```python
from build123d import *

# Parameters (mm, degrees)
F0_R      = 2.5
F1_DEPTH  = 2
F12_DEPTH = 2.0010001


with BuildPart() as f1:
    # F0 (on Top) → F1 (new body)
    with BuildSketch(Plane.XY):
        Polygon((-9.1669032276, 25.6), (-19.9169032276, 25.6), (-19.9169032276, 0), (-9.1669032276, 0), (-1.5169032276, 7.9), (30.5230967724, 7.9), (30.5230967724, 16.4), (2.6230967724, 16.4), (2.6230967724, 18.7), (-1.5169032276, 18.7), align=None)
        with Locations((-15.3946050969, 12.8)):
            Circle(F0_R, mode=Mode.SUBTRACT)
    extrude(amount=F1_DEPTH)

    # F4: sweep along a path in F2
    with BuildLine(Plane.XY.offset(2)) as f4_path:
        Line((2.6230967724, 15.15), (30.5230967724, 15.15))
    # F3 (on face) → F4 (sweep, cut)
    with BuildSketch(Plane.YZ.offset(2.6230967724)):
        with BuildLine():
            Line((17.3, 2), (15.3, 2))
            Line((15.3, 2), (14.7, 2))
            Line((14.7, 2), (15.5823529412, 0.75))
            add(Edge.make_bspline(
                [(15.5823529412, 0.75), (16.5972711165, 1.727867192), (16.3149181753, 1.727867192), (17.3, 2)],
                knots=[0, 0, 0, 0, 2.1243378777, 2.1243378777, 2.1243378777, 2.1243378777], degree=3))
        make_face()
    sweep(path=f4_path.line, mode=Mode.SUBTRACT)

    # F7: sweep along a path in F5
    with BuildLine(Plane.XY.offset(2)) as f7_path:
        Line((2.6230967724, 10.25), (30.5230967724, 10.25))
    # F6 (on face) → F7 (sweep, cut)
    with BuildSketch(Plane.YZ.offset(2.6230967724)):
        with BuildLine():
            add(Edge.make_bspline(
                [(11.55, 2), (11.1790336668, 1.9353309371), (10.4687979638, 0.1254777743), (8.7644318119, 0.7537172832), (8.7, 2)],
                knots=[0, 0, 0, 0, 0.4876224091, 1, 1, 1, 1], degree=3))
            Line((11.55, 2), (8.7, 2))
        make_face()
    sweep(path=f7_path.line, mode=Mode.SUBTRACT)

    # F10: sweep along a path in F8
    with BuildLine(Plane(origin=(0, 0, 0), x_dir=(1, 0, 0), z_dir=(0, 0, -1))) as f10_path:
        Line((2.6230967724, -17.2), (30.5230967724, -17.2))
    # F9 (on face) → F10 (sweep, cut)
    with BuildSketch(Plane.YZ.offset(2.6230967724)):
        with BuildLine():
            Line((17.2, 0), (17.2, 1))
            add(Edge.make_bspline(
                [(17.2, 1), (16.4, 1), (16.0935369316, 1.4085311701), (15.3480378536, 0.0682215952), (14.85, 0)],
                knots=[0, 0, 0, 0, 0.2283467357, 0.4887534963, 0.4887534963, 0.4887534963, 0.4887534963], degree=3))
            Line((14.85, 0), (17.2, 0))
        make_face()
        with BuildLine():
            Line((12.35, 0), (14.6790269663, 0))
            add(Edge.make_bspline(
                [(14.6790269663, 0), (14.1576409549, 0.0644703918), (13.0556896692, 1.1783434405), (12.4299004674, 0.6828821497), (12.35, 0)],
                knots=[0.5179423028, 0.5179423028, 0.5179423028, 0.5179423028, 0.7800763138, 1, 1, 1, 1], degree=3))
        make_face()
        with BuildLine():
            add(Edge.make_bspline(
                [(14.85, 0), (14.7941752951, -0.0076469096), (14.7370836655, -0.0071788235), (14.6790269663, 0)],
                knots=[0.4887534963, 0.4887534963, 0.4887534963, 0.4887534963, 0.5179423028, 0.5179423028, 0.5179423028, 0.5179423028], degree=3))
            Line((14.85, 0), (14.6790269663, 0))
        make_face()
    sweep(path=f10_path.line, mode=Mode.SUBTRACT)

    # F11 (on Top) → F12 (cut, through all)
    with BuildSketch(Plane.XY):
        Polygon((39.7434785501, 18.7), (2.6230967724, 18.7), (2.6230967724, 16.7), (5.3041512147, 16.7), (7.2075817734, 14.8422960192), (8.660200052, 14.8422960192), (10.6638120487, 16.5453646332), (12.7175133675, 16.5453646332), (15.0406220928, 14.2980599776), (16.7383030057, 14.2682762817), (19.5677690208, 16.4127144963), (24.6310271323, 16.3829308003), (25.3239014027, 15.8490902482), (30.2877575159, 12.3288799077), (30.4283164442, 11.5417372435), (25.4341885448, 7.3262052611), (39.7434785501, 7.5555583894), (39.7434785501, 11.2498085946), align=None)
    extrude(amount=F12_DEPTH, mode=Mode.SUBTRACT)


solid = f1.part
```
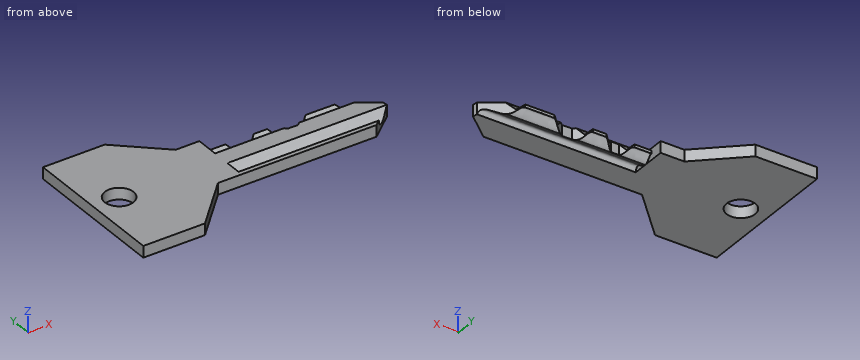
The model under review builds one solid part; all positions refer to its coordinate system, in mm. Round coordinates to 2 decimals unless told otherwise and drop trailing zeros. Loops run counter-clockwise (first coordinate to the right, second up) from the corner with the lowest first, then second, coordinate; pieces in that order, holes last. Notation, with made-up numbers: (10.5, 38.5) -> (26.5, 38.5) arc R15 cw to (26.5, 62.5) -> close; hole circle Ø2 at (14.25, 78). An arc over 180 degrees is marked (long way). Answer in a Markdown table with one row per item.
1) Wall thickness on line 1 along Y through (x, z) = (-15.5, 1.5); line 2 along Y through (x, z) = (22, 0.9); line 3 along X through (y, z) = (16.5, 0.2): over which ranges is each line inside the solid? List them lowest first.
Taken from the geometry:
| item | result |
|---|---|
| line 1 | y = 0 to 10.3, 15.3 to 25.6 |
| line 2 | y = 7.9 to 9.13, 10.47 to 15.48, 15.74 to 15.91 |
| line 3 | x = -19.92 to 2.62 |
2) Consider section B-B, the plane y = 5.75. Write out the cut boundary in (x, z), plus the area to 3 significant figures.
Taken from the geometry:
| item | result |
|---|---|
| outline | (-19.92, 0) -> (-3.6, 0) -> (-3.6, 2) -> (-19.92, 2) -> close |
| area | 32.6 mm² |
3) Consider section C-C, the plane x = -2.5. Write out the cut boundary in (y, z).
Taken from the geometry:
| item | result |
|---|---|
| outline | (6.88, 0) -> (19.59, 0) -> (19.59, 2) -> (6.88, 2) -> close |
4) Consider section A-A, the plane x = -16. Write out the cut boundary in (y, z).
Taken from the geometry:
| item | result |
|---|---|
| outline | (0, 0) -> (10.37, 0) -> (10.37, 2) -> (0, 2) -> close; (15.23, 0) -> (25.6, 0) -> (25.6, 2) -> (15.23, 2) -> close |
5) For pin 1 Ø1.2 at (x, z) = (7.5, 0.5) entering from +Y; pin 2 Ø1 at (x, y) = (24, 17.5) entering from +Z; pin 3 Ø10 at (x, y) = (20.5, 21) entering from -Z; pin 4 Ø1 at (x, z) = (2.5, 0.5) entering from -Y, all flat-tipped, find the tip position at first contact; note any pin that passes through.
Taken from the geometry:
| item | result |
|---|---|
| pin 1 | stops at y = 15.14 |
| pin 2 | passes through |
| pin 3 | stops at z = 0.99 |
| pin 4 | stops at y = 7.9 |
